Design review of the part built by this model. Coordinates are the model's own, in mm. Face numbers are marked on the shaded views. Give positions to 0.01 mm unless a question says otherwise; leave off trailing zeros. Loops run counter-clockwise (first coordinate to the right, second up) from the corner with the lowest first, then second, coordinate; pieces in that order, holes last. Notation, with made-up numbers: (16.5, -15.5) -> (75.5, -15.5) arc R18 cw to (75.5, -11.5) -> close; hole circle Ø3 at (-28.75, -7). An arc over 180 degrees is marked (long way). Use a Markdown table: item, result. Add a question column.
1. Draft analysis for pull direction X (two halves, no side actions). For the marked faces 1, 2, 3 and 4, state which applies: pulls with the +X half, pulls with the -X half, needs draft (parallel to the pull), parting line crosses it, or undercut.
2. Add section C-C (x = -116.5). State the section outline as (y, z) points.
3. To check wall thickness, follow line 1 (Y direction, x = 2, z = 2.5); line 2 (Y direction, x = 0, z = 11.5); line 3 (X direction, y = -82, z = 10). State the ranges of each line that lie inside material, in increasing order.
4. Add section D-D (z = 8.75). State the section outline as (x, y) points.
5. For pin 1 Ø1 at (x, y) = (50.5, -118) entering from -Z; pin 2 Ø6 at (x, z) = (-9, 12.5) entering from -Y; pin 3 Ø6 at (x, z) = (103.5, 4.5) entering from -Y; pin 4 Ø3 at (y, z) = (99.5, 14) entering from +X, all flat-tipped, find the tip position at first contact; note any pin that passes through.
6. Add section A-A (x = 0). State the section outline as (y, z) points.
7. Add section B-B (y = -106). State the section outline as (x, z) points.
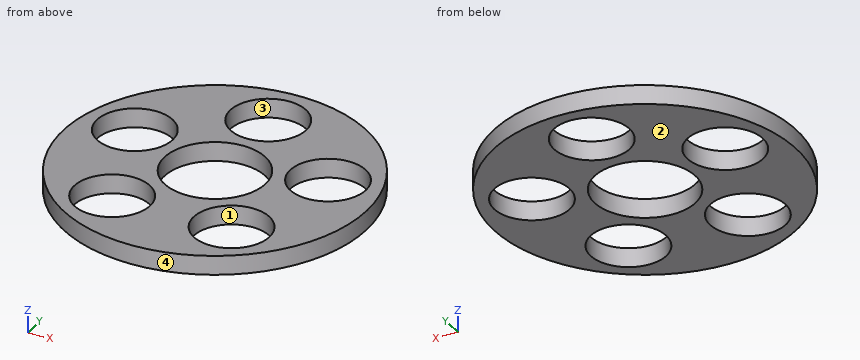
```python
from build123d import *

# Parameters (mm, degrees)
F0_R     = 150
F1_DEPTH = 19
F2_R     = 50
F2_R_2   = 37.5
F3_DEPTH = 53


with BuildPart() as f1:
    # F0 (on Top) → F1 (new body)
    with BuildSketch(Plane.XY):
        Circle(F0_R)
    extrude(amount=F1_DEPTH)

    # F2 (on face) → F3 (cut)
    with BuildSketch(Plane.XY.offset(19)):
        Circle(F2_R)
        with Locations((0, 100)):
            Circle(F2_R_2)
        with Locations((-95.105652, 30.901699)):
            Circle(F2_R_2)
        with Locations((-58.778525, -80.901699)):
            Circle(F2_R_2)
        with Locations((58.778525, -80.901699)):
            Circle(F2_R_2)
        with Locations((95.105652, 30.901699)):
            Circle(F2_R_2)
    extrude(amount=-F3_DEPTH, mode=Mode.SUBTRACT)


solid = f1.part
```
Taken from the geometry:
| question | item | result |
|---|---|---|
| 1 | face 1 | undercut |
| 1 | face 2 | needs draft |
| 1 | face 3 | undercut |
| 1 | face 4 | parting line crosses it |
| 2 | outline | (-94.49, 0) -> (0.1, 0) -> (0.1, 19) -> (-94.49, 19) -> close; (61.7, 0) -> (94.49, 0) -> (94.49, 19) -> (61.7, 19) -> close |
| 3 | line 1 | y = -149.99 to -49.96, 49.96 to 62.55, 137.45 to 149.99 |
| 3 | line 2 | y = -150 to -50, 50 to 62.5, 137.5 to 150 |
| 3 | line 3 | x = -125.6 to -96.26, -21.29 to 21.29, 96.26 to 125.6 |
| 4 | outline | circle Ø300 at (0, 0); hole circle Ø75 at (-95.11, 30.9); hole circle Ø75 at (-58.78, -80.9); hole circle Ø100 at (0, 0); hole circle Ø75 at (0, 100); hole circle Ø75 at (58.78, -80.9); hole circle Ø75 at (95.11, 30.9) |
| 5 | pin 1 | stops at z = 0 |
| 5 | pin 2 | stops at y = -149.88 |
| 5 | pin 3 | stops at y = -111.35 |
| 5 | pin 4 | stops at x = 113.56 |
| 6 | outline | (-150, 0) -> (-50, 0) -> (-50, 19) -> (-150, 19) -> close; (50, 0) -> (62.5, 0) -> (62.5, 19) -> (50, 19) -> close; (137.5, 0) -> (150, 0) -> (150, 19) -> (137.5, 19) -> close |
| 7 | outline | (-106.13, 0) -> (-86.64, 0) -> (-86.64, 19) -> (-106.13, 19) -> close; (-30.92, 0) -> (30.92, 0) -> (30.92, 19) -> (-30.92, 19) -> close; (86.64, 0) -> (106.13, 0) -> (106.13, 19) -> (86.64, 19) -> close |
